```python
from build123d import *

# Parameters (mm, degrees)
BOSS_EXTRUDE1_DEPTH      = 10
SKETCH3_W                = 74
SKETCH3_H                = 46
BOSS_EXTRUDE2_DEPTH      = 2
SKETCH4_R                = 1.25
CUT_EXTRUDE1_DEPTH       = 10
BOSS_EXTRUDE3_DEPTH      = 10
BOSS_EXTRUDE3_DEPTH_BACK = 2
SKETCH5_W                = 78
SKETCH5_H                = 50
SKETCH5_W_2              = 74
SKETCH5_H_2              = 46
SKETCH9_W                = 86.285123911
SKETCH9_H                = 6
SKETCH9_W_2              = 83.939508892
CUT_EXTRUDE2_DEPTH       = 10
FILLET1_R                = 3


with BuildPart() as part:
    # Sketch2 → Boss-Extrude1 (new body)
    with BuildSketch(Plane.XY):
        Polygon((-18.5, 0.5), (-18.5, -1), (-14.5, -1), (-14.5, -3.5), (-21.5, -3.5), (-21.5, -1), (-21.5, 3), (20.5, 3), (20.5, -3.5), (13.5, -3.5), (13.5, -1), (17.5, -1), (17.5, 0.5), align=None)
    extrude(amount=BOSS_EXTRUDE1_DEPTH)

    # Sketch3 → Boss-Extrude2 (add)
    with BuildSketch(Plane(origin=(0, 3, 0), x_dir=(1, 0, 0), z_dir=(0, 1, 0))):
        with Locations((1, -5)):
            Rectangle(SKETCH3_W, SKETCH3_H)
    extrude(amount=BOSS_EXTRUDE2_DEPTH)

    # Sketch4 → Cut-Extrude1 (cut)
    with BuildSketch(Plane(origin=(0, 5, 0), x_dir=(1, 0, 0), z_dir=(0, 1, 0))):
        with Locations(Location((-30, 10, 0), (0, 0, 180))):
            Circle(SKETCH4_R)
        with Locations(Location((-30, -20, 0), (0, 0, 180))):
            Circle(SKETCH4_R)
        with Locations(Location((32, 10, 0), (0, 0, 180))):
            Circle(SKETCH4_R)
        with Locations(Location((32, -20, 0), (0, 0, 180))):
            Circle(SKETCH4_R)
    extrude(amount=-CUT_EXTRUDE1_DEPTH, mode=Mode.SUBTRACT)

    # Sketch5 → Boss-Extrude3 (add, two sides: drawn at the far end of the back side and taken through both)
    with BuildSketch(Plane(origin=(0, 5, 0), x_dir=(1, 0, 0), z_dir=(0, 1, 0)).offset(-BOSS_EXTRUDE3_DEPTH_BACK)):
        with Locations((1, -5)):
            Rectangle(SKETCH5_W, SKETCH5_H)
        with Locations((1, -5)):
            Rectangle(SKETCH5_W_2, SKETCH5_H_2, mode=Mode.SUBTRACT)
    extrude(amount=BOSS_EXTRUDE3_DEPTH + BOSS_EXTRUDE3_DEPTH_BACK)

    # Sketch9 → Cut-Extrude2 (cut)
    with BuildSketch(Plane(origin=(0, 15, 0), x_dir=(1, 0, 0), z_dir=(0, 1, 0))):
        with Locations((1.40422043, 4)):
            Rectangle(SKETCH9_W, SKETCH9_H)
        with Locations((0.90158864, -14)):
            Rectangle(SKETCH9_W_2, SKETCH9_H)
    extrude(amount=-CUT_EXTRUDE2_DEPTH, mode=Mode.SUBTRACT)

    # Fillet1
    fillet1_edges = [part.edges().sort_by_distance(p)[0] for p in [
        (-37, 5, 17),
        (-37, 5, 11),
        (-37, 5, -7),
        (-37, 5, -1),
        (39, 5, 17),
        (39, 5, 11),
        (39, 5, -7),
        (39, 5, -1),
    ]]
    fillet(fillet1_edges, radius=FILLET1_R - 0.0001)  # a hair under: the kernel refuses the full size


solid = part.part
```
Source: CAD feature listing. Evaluate the final solid. Frame: model axes, mm. A direction names the side the tool comes from. Round coordinates to 2 decimals unless told otherwise and drop trailing zeros. Loops run counter-clockwise (first coordinate to the right, second up) from the corner with the lowest first, then second, coordinate; pieces in that order, holes last. Notation, with made-up numbers: M 32,-25 L 57,-25 A15 cw 57,-2 Z; hole C -11.75,38 d9. An arc over 180 degrees is marked long. Use a Markdown table: item, result. Add a question column.
1. Contact query for flat-ended pins moving along their axis: pin 1 (5 mm diameter, centred on x = 22, z = 9, fed in from +Y); pin 2 (3 mm diameter, centred on x = -30, z = 20, fed in from -Y); pin 3 (2 mm diameter, centred on x = 32, z = -10, fed in from -Y) (3 decimals); pin 4 (5 mm diameter, centred on x = 6.5, y = -1.5, fed in from +Z). Output: stop coordinate, or through.
2. Ray query, line 1 along Z through (x, y) = (32, 4); line 2 along Z through (x, y) = (-32.5, 5.25); line 3 along X through (y, z) = (9.25, 21). Return the intervals inside material, ascending. Write a range as [from, to].
3. Pull-direction query (Y, two-part tool) for faces 1 (the flat face through (0, 5, 5)), 2 (the flat face through (-14.5, -2, 5)), 3 (the flat face through (-17, -1, 5)); classes: +Y half, -Y half, draft (parallel to the pull), parting line (faces both ways), or undercut.
4. Cut plane B-B, the plane x = 32. Output: boundary loops of the cut face in (y, z), and give its area (3 significant figures).
5. Cut plane A-A, the plane y = 9.25. Output: boundary loops of the cut face in (x, z), and give its area (3 significant figures).
6. Cut plane D-D, the plane x = -8.5. Output: boundary loops of the cut face in (y, z), and give its area (3 significant figures).
7. Set-up query: faces 4 (the cylindrical face through (-36.99, 5.86, -1.9)), 5 (the flat face through (15, -1, 5)), 6 (the flat face through (-36, 10, 5)). Return all of +Z, -Z, +X, -X, +Y, -Y with unobstructed straight access to the full face (end or side cutting, diameter ignored); none if empty.
8. Cut plane C-C, the plane z = 20. Output: boundary loops of the cut face in (x, y), and give its area (3 significant figures).
Solution:
| question | item | result |
|---|---|---|
| 1 | pin 1 | stops at y = 5 |
| 1 | pin 2 | stops at y = 3 |
| 1 | pin 3 | passes through |
| 1 | pin 4 | stops at z = 10 |
| 2 | line 1 | z = [-20, -11.25], [-8.75, 18.75], [21.25, 30] |
| 2 | line 2 | z = [-20, -18], [28, 30] |
| 2 | line 3 | x = [-38, -36], [38, 40] |
| 3 | face 1 | +Y half |
| 3 | face 2 | draft |
| 3 | face 3 | undercut |
| 4 | outline | M 3,-20 L 15,-20 L 15,-18 L 5,-18 L 5,-11.25 L 3,-11.25 Z; M 3,-8.75 L 5,-8.75 L 5,18.75 L 3,18.75 Z; M 3,21.25 L 5,21.25 L 5,28 L 15,28 L 15,30 L 3,30 Z |
| 4 | area | 130 mm2 |
| 5 | outline | M -38,-20 L 40,-20 L 40,-7 L 38,-7 L 38,-18 L -36,-18 L -36,-7 L -38,-7 Z; M -38,-1 L -36,-1 L -36,11 L -38,11 Z; M -38,17 L -36,17 L -36,28 L 38,28 L 38,17 L 40,17 L 40,30 L -38,30 Z; M 38,-1 L 40,-1 L 40,11 L 38,11 Z |
| 5 | area | 448 mm2 |
| 6 | outline | M 0.5,0 L 3,0 L 3,-20 L 15,-20 L 15,-18 L 5,-18 L 5,28 L 15,28 L 15,30 L 3,30 L 3,10 L 0.5,10 Z |
| 6 | area | 165 mm2 |
| 7 | face 4 | +X, -X, +Y |
| 7 | face 5 | +Z, -Z |
| 7 | face 6 | +Y |
| 8 | outline | M -38,3 L -31.25,3 L -31.25,5 L -36,5 L -36,15 L -38,15 Z; M -28.75,3 L 30.75,3 L 30.75,5 L -28.75,5 Z; M 33.25,3 L 40,3 L 40,15 L 38,15 L 38,5 L 33.25,5 Z |
| 8 | area | 186 mm2 |
